from build123d import *

# Parameters (mm, degrees)
SKETCH1_R           = 101.5
SKETCH1_R_2         = 20
BOSS_EXTRUDE1_DEPTH = 75
SKETCH2_R           = 92.5
SKETCH2_R_2         = 27.5
CUT_EXTRUDE1_DEPTH  = 35
CUT_EXTRUDE2_START  = -35
SKETCH3_R           = 92.5
SKETCH3_R_2         = 27.5
CUT_EXTRUDE2_DEPTH  = 35


with BuildPart() as part:
    # Sketch1 → Boss-Extrude1 (new body)
    with BuildSketch(Plane.XY):
        Circle(SKETCH1_R)
        Circle(SKETCH1_R_2, mode=Mode.SUBTRACT)
        with BuildLine():
            Line((10, 80), (10, 40))
            ThreePointArc((10, 40), (0, 30), (-10, 40))
            Line((-10, 40), (-10, 80))
            ThreePointArc((-10, 80), (0, 90), (10, 80))
        make_face(mode=Mode.SUBTRACT)
        with BuildLine():
            Line((63.639610307, 49.497474683), (35.355339059, 21.213203436))
            ThreePointArc((35.355339059, 21.213203436), (21.213203436, 21.213203436), (21.213203436, 35.355339059))
            Line((21.213203436, 35.355339059), (49.497474683, 63.639610307))
            ThreePointArc((49.497474683, 63.639610307), (63.639610307, 63.639610307), (63.639610307, 49.497474683))
        make_face(mode=Mode.SUBTRACT)
        with BuildLine():
            Line((80, -10), (40, -10))
            ThreePointArc((40, -10), (30, 0), (40, 10))
            Line((40, 10), (80, 10))
            ThreePointArc((80, 10), (90, 0), (80, -10))
        make_face(mode=Mode.SUBTRACT)
        with BuildLine():
            Line((49.497474683, -63.639610307), (21.213203436, -35.355339059))
            ThreePointArc((21.213203436, -35.355339059), (21.213203436, -21.213203436), (35.355339059, -21.213203436))
            Line((35.355339059, -21.213203436), (63.639610307, -49.497474683))
            ThreePointArc((63.639610307, -49.497474683), (63.639610307, -63.639610307), (49.497474683, -63.639610307))
        make_face(mode=Mode.SUBTRACT)
        with BuildLine():
            Line((-10, -80), (-10, -40))
            ThreePointArc((-10, -40), (0, -30), (10, -40))
            Line((10, -40), (10, -80))
            ThreePointArc((10, -80), (0, -90), (-10, -80))
        make_face(mode=Mode.SUBTRACT)
        with BuildLine():
            Line((-63.639610307, -49.497474683), (-35.355339059, -21.213203436))
            ThreePointArc((-35.355339059, -21.213203436), (-21.213203436, -21.213203436), (-21.213203436, -35.355339059))
            Line((-21.213203436, -35.355339059), (-49.497474683, -63.639610307))
            ThreePointArc((-49.497474683, -63.639610307), (-63.639610307, -63.639610307), (-63.639610307, -49.497474683))
        make_face(mode=Mode.SUBTRACT)
        with BuildLine():
            Line((-80, 10), (-40, 10))
            ThreePointArc((-40, 10), (-30, 0), (-40, -10))
            Line((-40, -10), (-80, -10))
            ThreePointArc((-80, -10), (-90, 0), (-80, 10))
        make_face(mode=Mode.SUBTRACT)
        with BuildLine():
            Line((-49.497474683, 63.639610307), (-21.213203436, 35.355339059))
            ThreePointArc((-21.213203436, 35.355339059), (-21.213203436, 21.213203436), (-35.355339059, 21.213203436))
            Line((-35.355339059, 21.213203436), (-63.639610307, 49.497474683))
            ThreePointArc((-63.639610307, 49.497474683), (-63.639610307, 63.639610307), (-49.497474683, 63.639610307))
        make_face(mode=Mode.SUBTRACT)
    extrude(amount=BOSS_EXTRUDE1_DEPTH)

    # Sketch2 → Cut-Extrude1 (cut)
    with BuildSketch(Plane.XY.offset(75)):
        Circle(SKETCH2_R)
        Circle(SKETCH2_R_2, mode=Mode.SUBTRACT)
    extrude(amount=-CUT_EXTRUDE1_DEPTH, mode=Mode.SUBTRACT)

    # Sketch3 → Cut-Extrude2 (cut)
    with BuildSketch(Plane(origin=(0, 0, 0), x_dir=(-1, 0, 0), z_dir=(0, 0, -1)).offset(CUT_EXTRUDE2_START)):
        with Locations(Location((0, 0, 0), (0, 0, 180))):
            Circle(SKETCH3_R)
        with Locations(Location((0, 0, 0), (0, 0, 180))):
            Circle(SKETCH3_R_2, mode=Mode.SUBTRACT)
    extrude(amount=CUT_EXTRUDE2_DEPTH, mode=Mode.SUBTRACT)


solid = part.part
Could you check a few things on this model? Use its own coordinates, in mm. A direction names the side the tool comes from. Round coordinates to 2 decimals unless told otherwise and drop trailing zeros. Write each loop counter-clockwise with the first axis right and the second up, starting at its lowest first coordinate (ties: lowest second). Pieces come first, ordered by that corner, then holes. Notation, with made-up numbers: (78, 61) -> (82, 61) arc R26 ccw to (82, 82) -> close; hole circle Ø1 at (-37.5, -25.5). An arc over 180 degrees is marked (long way). Use a Markdown table: item, result.
1. Please list where these lines run through material, in increasing order: probe 1 along Y at (x, z) = (0, 65); probe 2 along Y at (x, z) = (0, 38); probe 3 along X at (y, z) = (-14, 46.5).
Answer key:
| item | result |
|---|---|
| probe 1 | y = -101.5 to -92.5, -27.5 to -20, 20 to 27.5, 92.5 to 101.5 |
| probe 2 | y = -101.5 to -90, -30 to -20, 20 to 30, 90 to 101.5 |
| probe 3 | x = -100.53 to -91.43, -23.67 to -14.28, 14.28 to 23.67, 91.43 to 100.53 |
2. If we section it at A-A (y = 0): State how many separate pieces and enclosed holes the cut face has, then the cut area to 4 significant figures.
Answer key:
| item | result |
|---|---|
| separate pieces | 4 |
| enclosed holes | 0 |
| area | 2,525 mm^2 |
3. If we section it at B-B (x = -69): List the corners of the cut face in (y, z) for me, then the cut area to 3 significant figures.
Answer key:
| item | result |
|---|---|
| outline | (-74.44, 0) -> (-61.61, 0) -> (-61.61, 35) -> (-10, 35) -> (-10, 40) -> (-61.61, 40) -> (-61.61, 75) -> (-74.44, 75) -> close; (10, 35) -> (61.61, 35) -> (61.61, 0) -> (74.44, 0) -> (74.44, 75) -> (61.61, 75) -> (61.61, 40) -> (10, 40) -> close |
| area | 2,440 mm^2 |
4. Which directions (+Z, -Z, +X, -X, +Y, -Y) give clear straight access to the entire face, cutting with the end or side of a thin tool? Please do faces 4 (the face through (-22, -19, 40)), 5 (the face through (12.69, 24.397, 17.745)), 6 (the face through (30, 0, 37)), 7 (the face through (1.9, -20.2, 0)).
Answer key:
| item | result |
|---|---|
| face 4 | +Z |
| face 5 | -Z |
| face 6 | +Z, -Z |
| face 7 | -Z, +X, -X, +Y, -Y |
5. For pin 1 Ø5 at (x, z) = (-50.5, 17.5) entering from -Y; pin 2 Ø2.5 at (y, z) = (50.5, 38.5) entering from -X; pin 3 Ø5 at (x, y) = (10.5, 35.5) entering from -Z, each with a flat end and sliding along its axis, tell me the tip position at first contact or that it passes through.
Answer key:
| item | result |
|---|---|
| pin 1 | stops at y = -89.43 |
| pin 2 | stops at x = -88.75 |
| pin 3 | stops at z = 35 |
6. If we section it at D-D (y = 57): List the corners of the cut face in (x, z) for me, then the cut area to 3 significant figures.
Answer key:
| item | result |
|---|---|
| outline | (-83.98, 0) -> (-72.85, 0) -> (-72.85, 35) -> (-66.56, 35) -> (-66.56, 40) -> (-72.85, 40) -> (-72.85, 75) -> (-83.98, 75) -> close; (-42.86, 35) -> (-10, 35) -> (-10, 40) -> (-42.86, 40) -> close; (10, 35) -> (42.86, 35) -> (42.86, 40) -> (10, 40) -> close; (66.56, 35) -> (72.85, 35) -> (72.85, 0) -> (83.98, 0) -> (83.98, 75) -> (72.85, 75) -> (72.85, 40) -> (66.56, 40) -> close |
| area | 2,060 mm^2 |
7. If we section it at C-C (x = 56): List the corners of the cut face in (y, z) for me, then the cut area to 3 significant figures.
Answer key:
| item | result |
|---|---|
| outline | (-84.65, 0) -> (-73.62, 0) -> (-73.62, 35) -> (-66.55, 35) -> (-66.55, 40) -> (-73.62, 40) -> (-73.62, 75) -> (-84.65, 75) -> close; (-41.86, 35) -> (-10, 35) -> (-10, 40) -> (-41.86, 40) -> close; (10, 35) -> (41.86, 35) -> (41.86, 40) -> (10, 40) -> close; (66.55, 35) -> (73.62, 35) -> (73.62, 0) -> (84.65, 0) -> (84.65, 75) -> (73.62, 75) -> (73.62, 40) -> (66.55, 40) -> close |
| area | 2,040 mm^2 |
8. We'd pull the mould along X, two halves only. Please class faces 1 (the face through (96.813, 30.488, 36.975)), 2 (the face through (90, 23, 0)), 3 (the face through (35.553, -49.695, 37.465)): +X half, -X half, draft (parallel to the pull), parting line (faces both ways), or undercut.
Answer key:
| item | result |
|---|---|
| face 1 | parting line |
| face 2 | draft |
| face 3 | undercut |
